For this review, take the finished solid that the model builds, in its own axes (mm). Face numbers are marked on the shaded views. A direction names the side the tool comes from. Round coordinates to 2 decimals unless told otherwise and drop trailing zeros. Order: outer loops, then holes, each group sorted by start corner. A loop starts at its lowest first (then second) coordinate and runs counter-clockwise, first axis right, second up. Notation, with made-up numbers: (-15, -9.5) -> (35, -9.5) arc R21 ccw to (35, 6.5) -> close; hole circle Ø6 at (-30.75, 57). An arc over 180 degrees is marked (long way). Use a Markdown table: item, result. Add a question column.
1) Wall thickness on line 1 along Z through (x, y) = (19, -16); line 2 along X through (y, z) = (-24, -30); line 3 along Z through (x, y) = (31, -30): over which ranges is each line inside the solid? List them lowest first. Write a range as [from, to].
2) Draft analysis for pull direction Z (two halves, no side actions). For the marked faces 1, 2 and 3, state which applies: pulls with the +Z half, pulls with the -Z half, needs draft (parallel to the pull), parting line crosses it, or undercut.
3) Clearance check with flat-ended pins moving along their axes: P1, Ø4.5, axis at y = 17.63, z = -30.53, coming from the +X side; P2, Ø5, axis at y = -26.5, z = 54.5, coming from the -X side; P3, Ø12, axis at y = 12, z = -55, coming from the +X side. State where each tip first meets the part, or that it passes through.
4) Machinability: for the marked faces 4, 5, 6, 7 and 8, which of the approach directions +Z, -Z, +X, -X, +Y, -Y give a long, thin tool a straight path to every point of the face, cutting with its end or side? Answer none if there is none.
5) Consider section D-D (x = 47.5). State the section outline as (y, z) points.
6) Consider section C-C (z = 39.5). State the section outline as (x, y) points.
7) Consider section A-A (y = -57.09). State the section outline as (x, z) points (3 decimals).
8) Consider section B-B (x = 32). State the section outline as (y, z) points (3 decimals), plus the area to 3 significant figures.
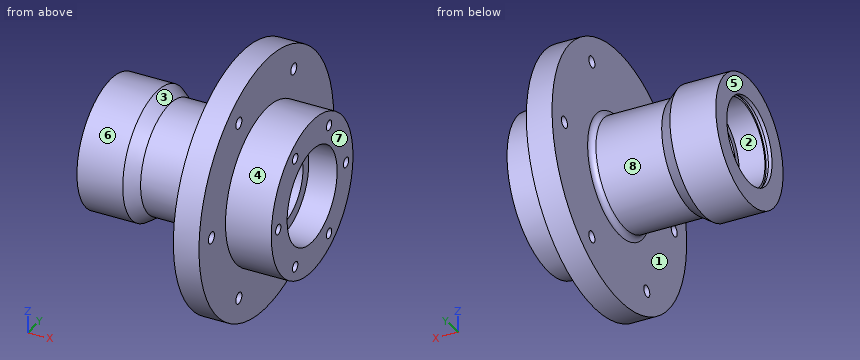
```python
from build123d import *

# Parameters (mm, degrees)
SCHIZZO2_R                  = 3.125
TAGLIO_ESTRUSIONE1_DEPTH    = 14
RIPETIZIONECIRCOLARE1_COUNT = 6
RACCORDO1_R                 = 3


with BuildPart() as part:
    # Schizzo1 → Rivoluzione1 (revolve)
    with BuildSketch(Plane.XY):
        Polygon((-41.225471698, 23.5), (-27.225471698, 23.5), (-27.225471698, 20), (49.424528302, 20), (49.424528302, 26), (64.924528302, 26), (64.924528302, 42.5), (39.924528302, 42.5), (39.924528302, 70), (25.924528302, 70), (25.924528302, 30), (-12.934731664, 30), (-20.075471698, 35), (-45.075471698, 35), (-45.075471698, 23.5), (-43.075471698, 23.5), (-43.075471698, 24.75), (-41.225471698, 24.75), align=None)
    revolve(axis=Axis((0, 0, 0), (1, 0, 0)))

    # Schizzo2 → Taglio-Estrusione1 (cut)
    with BuildSketch(Plane(origin=(39.924528302, 0, 0), x_dir=(0, 0, -1), z_dir=(1, 0, 0))):
        with Locations((0, 57.09)):
            Circle(SCHIZZO2_R)
    taglio_estrusione1 = extrude(amount=-TAGLIO_ESTRUSIONE1_DEPTH, mode=Mode.SUBTRACT)

    # Schizzo5 → Foro per Vite M5-1 (revolve, cut)
    with BuildSketch(Plane(origin=(64.924528302, 35.25, 0), x_dir=(0, 0, -1), z_dir=(0, 1, 0))):
        Polygon((0, 0), (0, 12), (2.75, 10.347633298), (2.75, 0), align=None)
    foro_per_vite_m5_1 = revolve(axis=Axis((71.274528302, 35.25, 0), (-1, 0, 0)), mode=Mode.SUBTRACT)

    # RipetizioneCircolare1: Taglio-Estrusione1, Foro per Vite M5-1 ×6 about axis
    ripetizionecircolare1_axis = Axis((0, 0, 0), (1, 0, 0))
    for i in range(1, RIPETIZIONECIRCOLARE1_COUNT):
        add(taglio_estrusione1.rotate(ripetizionecircolare1_axis, i * 360 / RIPETIZIONECIRCOLARE1_COUNT), mode=Mode.SUBTRACT)
        add(foro_per_vite_m5_1.rotate(ripetizionecircolare1_axis, i * 360 / RIPETIZIONECIRCOLARE1_COUNT), mode=Mode.SUBTRACT)

    # Raccordo1
    raccordo1_edges = [part.edges().sort_by_distance(p)[0] for p in [
        (25.924528302, -30, 0),
    ]]
    fillet(raccordo1_edges, radius=RACCORDO1_R)


solid = part.part
```
Results list:
| question | item | result |
|---|---|---|
| 1 | line 1 | [-25.38, -12], [12, 25.38] |
| 1 | line 2 | [25.92, 64.92] |
| 1 | line 3 | [-63.25, -52.21], [-46.68, 46.68], [52.21, 63.25] |
| 2 | face 1 | needs draft |
| 2 | face 2 | undercut |
| 2 | face 3 | parting line crosses it |
| 3 | P1 | x = 54.28 |
| 3 | P2 | x = 25.92 |
| 3 | P3 | x = 39.92 |
| 4 | face 4 | +X |
| 4 | face 5 | +Z, -Z, -X, +Y, -Y |
| 4 | face 6 | -X |
| 4 | face 7 | +Z, -Z, +X, +Y, -Y |
| 4 | face 8 | none |
| 5 | outline | circle Ø85 at (0, 0); hole circle Ø40 at (0, 0) |
| 6 | outline | (25.92, -57.79) -> (39.92, -57.79) -> (39.92, -15.68) -> (64.92, -15.68) -> (64.92, 15.68) -> (39.92, 15.68) -> (39.92, 57.79) -> (25.92, 57.79) -> close |
| 7 | outline | (25.925, -40.506) -> (39.925, -40.506) -> (39.925, -3.125) -> (25.925, -3.125) -> close; (25.925, 3.125) -> (39.925, 3.125) -> (39.925, 40.506) -> (25.925, 40.506) -> close |
| 8 | outline | circle Ø140 at (0, 0); hole circle Ø6.25 at (-57.09, 0); hole circle Ø6.25 at (-28.545, -49.441); hole circle Ø6.25 at (-28.545, 49.441); hole circle Ø40 at (0, 0); hole circle Ø6.25 at (28.545, -49.441); hole circle Ø6.25 at (28.545, 49.441); hole circle Ø6.25 at (57.09, 0) |
| 8 | area | 14,000 mm2 |
